Build history of the part. All positions in model axes, mm. Face numbers are marked on the shaded views. A direction names the side the tool comes from. Give positions to 0.01 mm unless a question says otherwise; leave off trailing zeros. Loops run counter-clockwise (first coordinate to the right, second up) from the corner with the lowest first, then second, coordinate; pieces in that order, holes last. Notation, with made-up numbers: (48, 37) - (67, 37) arc R19 cw to (67, 48) - close; hole circle Ø8 at (2, 42.5). An arc over 180 degrees is marked (long way). Return JSON: item names as keys, results as strings. Group by question number.
1) Slice it at C-C (y = 0). List the corners of the cut face in (x, z).
2) Slice it at D-D (x = -14). List the corners of the cut face in (y, z), and give its area (3 significant figures).
3) Drop flat-ended pins along their axis: pin 1 (1.5 mm diameter, centred on x = 2, z = 21, fed in from -Y); pin 2 (9 mm diameter, centred on x = 42, y = 0, fed in from -Z); pin 3 (10 mm diameter, centred on x = -6, z = 16.5, fed in from +Y); pin 4 (10 mm diameter, centred on y = 12.5, z = 4, fed in from -X). Give the stop position or say it passes through.
4) Slice it at A-A (x = 0). List the corners of the cut face in (y, z), and give its area (3 significant figures).
5) Drill centre lines: probe 1 along X at (y, z) = (-0.5, 8.5); probe 2 along Y at (x, z) = (0, 21.25); probe 3 along Y at (x, z) = (4, 24). Where is each one in solid material? Low to high. Write a range as from..to.
6) Slice it at B-B (z = 7). List the corners of the cut face in (x, y).
7) 3-axis set-ups, long thin cutter, end or side, ignore diameter. For the marked faces 1 and 2: which of +Z, -Z, +X, -X, +Y, -Y reach the whole face in a straight line?
8) Mould opens along Y. For the marked faces 3, 4, 5 and 6 say: released by +Y, released by -Y, zero draft, split by the parting line, or undercut.
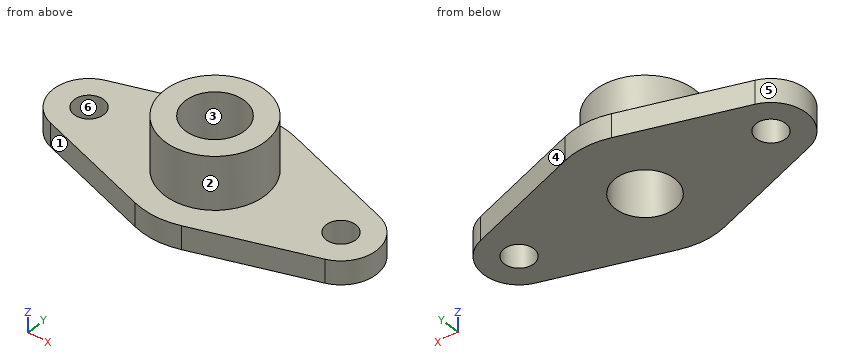
```python
from build123d import *

# Parameters (mm, degrees)
EXTRUDE_1_DEPTH     = 8
SKETCH_2_R          = 17
EXTRUDE_2_DEPTH     = 18
SKETCH_3_R          = 10
CUT_EXTRUDE_1_DEPTH = 65.93843238
SKETCH_4_R          = 5
CUT_EXTRUDE_2_DEPTH = 65.93843238


with BuildPart() as part:
    # 草图1 → 凸台-拉伸1 (new body)
    with BuildSketch(Plane.XY):
        with BuildLine():
            Line((-7.738095, 23.7723), (-45.714286, 11.410704))
            ThreePointArc((-45.714286, 11.410704), (-54, 0), (-45.714286, -11.410704))
            Line((-45.714286, -11.410704), (-7.738095, -23.7723))
            ThreePointArc((-7.738095, -23.7723), (0, -25), (7.738095, -23.7723))
            Line((7.738095, -23.7723), (45.714286, -11.410704))
            ThreePointArc((45.714286, -11.410704), (54, 0), (45.714286, 11.410704))
            Line((45.714286, 11.410704), (7.738095, 23.7723))
            ThreePointArc((7.738095, 23.7723), (0, 25), (-7.738095, 23.7723))
        make_face()
    extrude(amount=EXTRUDE_1_DEPTH)

    # 草图2 → 凸台-拉伸2 (add)
    with BuildSketch(Plane.XY.offset(8)):
        Circle(SKETCH_2_R)
    extrude(amount=EXTRUDE_2_DEPTH)

    # 草图3 → 切除-拉伸1 (cut, through all)
    with BuildSketch(Plane.XY):
        with Locations(Location((0, 0, 0), (0, 0, 180))):
            Circle(SKETCH_3_R)
    extrude(amount=CUT_EXTRUDE_1_DEPTH, mode=Mode.SUBTRACT)

    # 草图4 → 切除-拉伸2 (cut, through all)
    with BuildSketch(Plane.XY):
        with Locations(Location((42, 0, 0), (0, 0, 180))):
            Circle(SKETCH_4_R)
        with Locations(Location((-42, 0, 0), (0, 0, 180))):
            Circle(SKETCH_4_R)
    extrude(amount=CUT_EXTRUDE_2_DEPTH, mode=Mode.SUBTRACT)


solid = part.part
```
Results:
{
 "1": {"outline": "(-54, 0) - (-47, 0) - (-47, 8) - (-54, 8) - close; (-37, 0) - (-10, 0) - (-10, 26) - (-17, 26) - (-17, 8) - (-37, 8) - close; (10, 0) - (37, 0) - (37, 8) - (17, 8) - (17, 26) - (10, 26) - close; (47, 0) - (54, 0) - (54, 8) - (47, 8) - close"},
 "2": {"outline": "(-21.73, 0) - (21.73, 0) - (21.73, 8) - (9.64, 8) - (9.64, 26) - (-9.64, 26) - (-9.64, 8) - (-21.73, 8) - close", "area": "695 mm2"},
 "3": {"pin 1": "y = -16.95", "pin 2": "through", "pin 3": "y = 16.97", "pin 4": "x = -51.37"},
 "4": {"outline": "(-25, 0) - (-10, 0) - (-10, 26) - (-17, 26) - (-17, 8) - (-25, 8) - close; (10, 0) - (25, 0) - (25, 8) - (17, 8) - (17, 26) - (10, 26) - close", "area": "492 mm2"},
 "5": {"probe 1": "-16.99..-9.99, 9.99..16.99", "probe 2": "-17..-10, 10..17", "probe 3": "-16.52..-9.17, 9.17..16.52"},
 "6": {"outline": "(-45.71, -11.41) - (-7.74, -23.77) arc R25 ccw to (7.74, -23.77) - (45.71, -11.41) arc R12 ccw to (45.71, 11.41) - (7.74, 23.77) arc R25 ccw to (-7.74, 23.77) - (-45.71, 11.41) arc R12 ccw to start; hole circle Ø10 at (-42, 0); hole circle Ø20 at (0, 0); hole circle Ø10 at (42, 0)"},
 "7": {"face 1": "+Z, -Z, -X, -Y", "face 2": "+Z"},
 "8": {"face 3": "undercut", "face 4": "released by +Y", "face 5": "split by the parting line", "face 6": "undercut"}
}
